from build123d import *

# Parameters (mm, degrees)
SKETCH1_W           = 57.15
SKETCH1_H           = 5.08
BOSS_EXTRUDE1_DEPTH = 152.4
CUT_EXTRUDE1_DEPTH  = 1
SKETCH3_W           = 57.15
SKETCH3_H           = 5.08
BOSS_EXTRUDE2_DEPTH = 12.7
SKETCH4_R           = 2.25
CUT_EXTRUDE2_DEPTH  = 12.7


with BuildPart() as part:
    # Sketch1 → Boss-Extrude1 (new body)
    with BuildSketch(Plane(origin=(0, 0, 0), x_dir=(1, 0, 0), z_dir=(0, 1, 0))):
        Rectangle(SKETCH1_W, SKETCH1_H)
    extrude(amount=-BOSS_EXTRUDE1_DEPTH)

    # Sketch2 → Cut-Extrude1 (cut)
    with BuildSketch(Plane.XY.offset(2.54)):
        Polygon((-5.125, -152.4), (-5.125, -50.8), (5.125, -50.8), (5.125, -152.4), (28.575, -152.4), (28.575, -12.7), (-28.575, -12.7), (-28.575, -152.4), align=None)
    extrude(amount=-CUT_EXTRUDE1_DEPTH, mode=Mode.SUBTRACT)

    # Sketch3 → Boss-Extrude2 (add)
    with BuildSketch(Plane(origin=(0, 0, -2.54), x_dir=(-1, 0, 0), z_dir=(0, 0, -1))):
        with Locations((0, -2.54)):
            Rectangle(SKETCH3_W, SKETCH3_H)
    extrude(amount=BOSS_EXTRUDE2_DEPTH)

    # Sketch4 → Cut-Extrude2 (cut)
    with BuildSketch(Plane(origin=(0, 0, 0), x_dir=(1, 0, 0), z_dir=(0, 1, 0))):
        with Locations(Location((0, 10.16, 0), (0, 0, 270))):
            Circle(SKETCH4_R)
    extrude(amount=-CUT_EXTRUDE2_DEPTH, mode=Mode.SUBTRACT)


solid = part.part
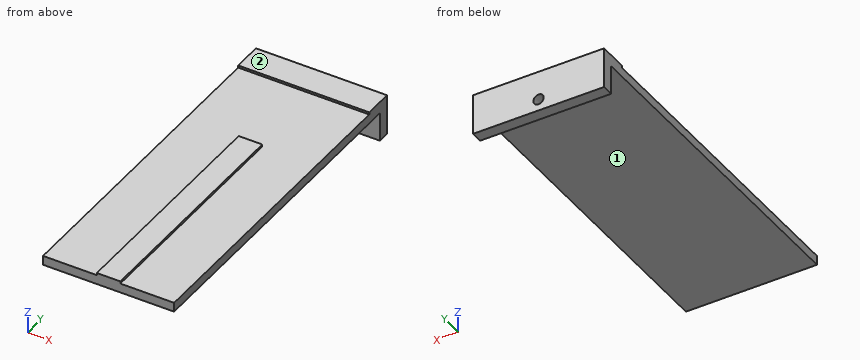
The listing builds one solid part. Answer for the finished solid, in the listing's coordinates (mm). Face numbers are marked on the shaded views. A direction names the side the tool comes from. Give positions to 0.01 mm unless a question says otherwise; leave off trailing zeros. Loops run counter-clockwise (first coordinate to the right, second up) from the corner with the lowest first, then second, coordinate; pieces in that order, holes last.
Item 1: A cutting plane is placed at A-A (x = 0). Give the vertices of the cut face in (y, z).
Derived:
outline: (-152.4, -2.54) - (-5.08, -2.54) - (-5.08, -7.91) - (0, -7.91) - (0, 2.54) - (-12.7, 2.54) - (-12.7, 1.54) - (-50.8, 1.54) - (-50.8, 2.54) - (-152.4, 2.54) - close; (-5.08, -15.24) - (0, -15.24) - (0, -12.41) - (-5.08, -12.41) - close
Item 2: A cutting plane is placed at B-B (z = -10.16). Give the vertices of the cut face in (x, y) (3 decimals), then the cut area to 3 significant figures.
Derived:
outline: (-28.575, -5.08) - (-2.25, -5.08) - (-2.25, 0) - (-28.575, 0) - close; (2.25, -5.08) - (28.575, -5.08) - (28.575, 0) - (2.25, 0) - close
area: 267 mm2
Item 3: A cutting plane is placed at C-C (y = -62). Give the vertices of the cut face in (x, z) (3 decimals), then the cut area to 3 significant figures.
Derived:
outline: (-28.575, -2.54) - (28.575, -2.54) - (28.575, 1.54) - (5.125, 1.54) - (5.125, 2.54) - (-5.125, 2.54) - (-5.125, 1.54) - (-28.575, 1.54) - close
area: 243 mm2
Item 4: Each of these flat-tipped pins is pushed along its axis until it touches: pin 1 Ø0.5 at (x, z) = (-7, 2) entering from -Y; pin 2 Ø10 at (x, z) = (-7.5, -11.5) entering from -Y; pin 3 Ø4 at (x, z) = (0, -10.16) entering from -Y; pin 4 Ø8 at (x, y) = (10.5, -109) entering from +Z. Where does it stop, or does it pass through?
Derived:
pin 1: stops at y = -12.7
pin 2: stops at y = -5.08
pin 3: passes through
pin 4: stops at z = 1.54
Item 5: A tool of negligible diameter and unlimited length cuts with its end or side. For the marked faces 1 and 2, from which of +Z, -Z, +X, -X, +Y, -Y can it reach the whole face along a straight path? Write none if from no direction.
Derived:
face 1: -Z, +X, -X, -Y
face 2: +Z, +X, -X, +Y, -Y
Item 6: Find the intervals of material crossed by line 1 along X through (y, z) = (-1.75, -10.16) (3 decimals); line 2 along Z through (x, y) = (-12.5, -60.5); line 3 along Y through (x, z) = (14, -7.75), in increasing order.
Derived:
line 1: x = -28.575 to -2.25, 2.25 to 28.575
line 2: z = -2.54 to 1.54
line 3: y = -5.08 to 0
Item 7: A cutting plane is placed at D-D (x = -22). Give the vertices of the cut face in (y, z), then the cut area to 3 significant figures.
Derived:
outline: (-152.4, -2.54) - (-5.08, -2.54) - (-5.08, -15.24) - (0, -15.24) - (0, 2.54) - (-12.7, 2.54) - (-12.7, 1.54) - (-152.4, 1.54) - close
area: 699 mm2
